Part model, mm, in its own coordinate system. Face numbers are marked on the shaded views. Round coordinates to 2 decimals unless told otherwise and drop trailing zeros. Order: outer loops, then holes, each group sorted by start corner. A loop starts at its lowest first (then second) coordinate and runs counter-clockwise, first axis right, second up. Notation, with made-up numbers: M -25,-31.75 L 10,-31.75 A28 cw 10,-5.75 Z; hole C 3,-23 d2. An arc over 180 degrees is marked long. Write each question's results on one line, items separated by ' | '. Start each with the question number.
1. Drop flat-ended pins along their axis: pin 1 Ø16 at (x, y) = (31.5, 37) entering from +Z; pin 2 Ø10.5 at (x, y) = (0, 57) entering from -Z; pin 3 Ø5 at (y, z) = (50.5, 1.5) entering from -X. Give the stop position or say it passes through.
2. Two-plate mould, pull along X, no slides. Class the marked faces 1, 2 and 3: +X half, -X half, draft (parallel to the pull), parting line (faces both ways), or undercut.
3. Probe L1, parallel to Y at x = 42.5, z = 7; L2, parallel to Y at x = 0, z = 4.4; L3, parallel to X at y = 57, z = 4.1. List the from-to ranges inside material, lowest first. Write a range as [from, to].
4. Band-saw the part on A-A, the plane z = 9.5. List the corners of the cut face in (x, y).
5. Band-saw the part on B-B, the plane x = 1.5. List the corners of the cut face in (y, z), then the cut area to 3 significant figures.
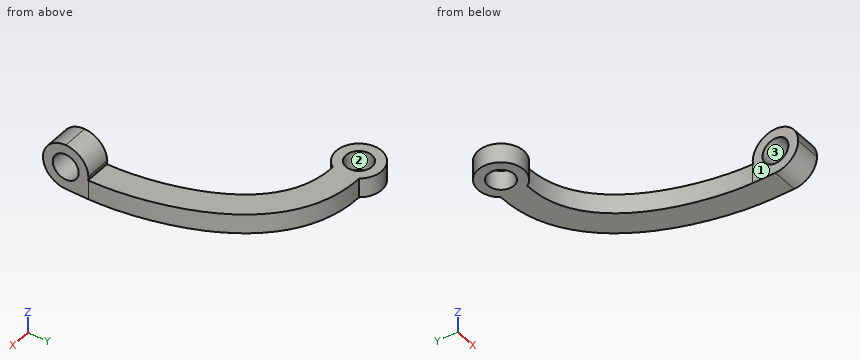
```python
from build123d import *
from OCP.BRepAlgoAPI import BRepAlgoAPI_Cut
from OCP.TopTools import TopTools_ListOfShape

# Parameters (mm, degrees)
ESBO_O1_R                = 4
RESSALTO_EXTRUS_O1_DEPTH = 14
ESBO_O2_R                = 4
CORTE_EXTRUS_O1_DEPTH    = 85.267431587


with BuildPart() as part:
    # Esboço1 → Ressalto-extrusão1 (new body)
    with BuildSketch(Plane.XY):
        with BuildLine():
            Line((46, -7), (46, 6.995688759))
            add(Edge.make_bspline(
                [(5.650259544, 61.132138319), (6.660650147, 61.155575151), (8.710848107, 61.120789853), (12.578892548, 60.727605083), (17.127930578, 59.655790613), (22.040205616, 57.539349047), (26.394344624, 54.722364625), (30.19261077, 51.343572081), (34.558581899, 46.260896731), (38.815468688, 39.112541001), (41.760696394, 31.545459809), (43.470535674, 25.587286464), (44.459557745, 21.252306014), (45.183880004, 17.135758602), (45.589217997, 13.957943213), (45.8071763, 11.605329402), (45.920450747, 9.949575993), (45.986308659, 8.391657602), (46.000256085, 7.470883976), (46, 6.995688759)],
                knots=[0, 0, 0, 0, 0.03125, 0.0625, 0.125, 0.1875, 0.25, 0.3125, 0.375, 0.5, 0.625, 0.6875, 0.75, 0.8125, 0.875, 0.90625, 0.9375, 0.96875, 1, 1, 1, 1], degree=3))
            ThreePointArc((5.650259544, 61.132138319), (-6.998117599, 56.837672963), (5.835776158, 53.134289634))
            add(Edge.make_bspline(
                [(5.835776158, 53.134289634), (6.238188643, 53.143623919), (7.052270041, 53.146185942), (8.608930463, 53.086843267), (10.474039614, 52.897553491), (12.577068171, 52.49932445), (15.220765339, 51.755589596), (18.249448664, 50.451415), (21.515264324, 48.342822315), (24.453790354, 45.735335437), (27.957095233, 41.667286815), (31.567422767, 35.644835437), (34.179252288, 28.956801958), (35.718249768, 23.595597215), (36.614783762, 19.667281612), (37.272272941, 15.930397286), (37.638098577, 13.059067768), (37.83252613, 10.960084825), (37.932188748, 9.497611194), (37.979377076, 8.387903873), (37.997359238, 7.565341164), (38.000104404, 7.191578727), (38.000001162, 7)],
                knots=[0, 0, 0, 0, 0.015625, 0.03125, 0.0625, 0.09375, 0.125, 0.1875, 0.25, 0.3125, 0.375, 0.5, 0.625, 0.6875, 0.75, 0.8125, 0.875, 0.90625, 0.9375, 0.96875, 0.984375, 1, 1, 1, 1], degree=3))
            Line((38.000001162, 7), (38.000001162, -7))
            Line((38.000001162, -7), (46, -7))
        make_face()
        with Locations((0, 57)):
            Circle(ESBO_O1_R, mode=Mode.SUBTRACT)
    extrude(amount=RESSALTO_EXTRUS_O1_DEPTH)


with BuildPart() as corte_extrus_o1_tool:
    # Esboço2 → Corte-extrusão1 (new, through all)
    with BuildSketch(Plane(origin=(46, 0, 0), x_dir=(0, 0, -1), z_dir=(1, 0, 0))):
        with BuildLine():
            ThreePointArc((-7, -7), (-11.949747468, -4.949747468), (-14, 0))
            Line((-14, 0), (-14, -7))
            Line((-14, -7), (-7, -7))
        make_face()
        with BuildLine():
            Line((-7.245639543, 6.995688759), (-14, 6.995688759))
            Line((-14, 6.995688759), (-14, 0))
            ThreePointArc((-14, 0), (-12.035845351, 4.862125214), (-7.245639543, 6.995688759))
        make_face()
        with Locations((-7, 0)):
            Circle(ESBO_O2_R)
        with BuildLine():
            Line((0, -7), (0, 0))
            ThreePointArc((0, 0), (-2.050252532, -4.949747468), (-7, -7))
            Line((-7, -7), (0, -7))
        make_face()
        with BuildLine():
            Line((-6, 6.92820323), (-6, 6.995688759))
            Line((-6, 6.995688759), (-6.754360457, 6.995688759))
            ThreePointArc((-6.754360457, 6.995688759), (-6.37626685, 6.972155833), (-6, 6.92820323))
        make_face()
        with BuildLine():
            Line((-6, 6.995688759), (-6, 64))
            Line((-6, 64), (-14, 64))
            Line((-14, 64), (-14, 6.995688759))
            Line((-14, 6.995688759), (-7.245639543, 6.995688759))
            ThreePointArc((-7.245639543, 6.995688759), (-7, 7), (-6.754360457, 6.995688759))
            Line((-6.754360457, 6.995688759), (-6, 6.995688759))
        make_face()
    extrude(amount=-CORTE_EXTRUS_O1_DEPTH)


with BuildPart() as part_1:
    add(part.part)

    # Corte-extrusão1: cut by corte_extrus_o1_tool, with a tolerance
    corte_extrus_o1_stock = TopTools_ListOfShape()
    corte_extrus_o1_stock.Append(part_1.part.wrapped)
    corte_extrus_o1_tools = TopTools_ListOfShape()
    corte_extrus_o1_tools.Append(corte_extrus_o1_tool.part.wrapped)
    corte_extrus_o1_cut = BRepAlgoAPI_Cut()
    corte_extrus_o1_cut.SetArguments(corte_extrus_o1_stock)
    corte_extrus_o1_cut.SetTools(corte_extrus_o1_tools)
    corte_extrus_o1_cut.SetFuzzyValue(0.00001)
    corte_extrus_o1_cut.Build()
    add(Compound.cast(corte_extrus_o1_cut.Shape()).solids(), mode=Mode.REPLACE)


with BuildPart() as corte_extrus_o1_kept_piece:
    # of the separate pieces the step leaves, the one the design keeps (corte_extrus_o1_pieces_kept)
    add(part_1.part.solids().sort_by_distance((46, 0, 0))[0])


solid = corte_extrus_o1_kept_piece.part
```
Solution:
1) pin 1: z = 6 | pin 2: z = 0 | pin 3: x = -5.74
2) face 1: -X half | face 2: undercut | face 3: draft
3) L1: [-7, -4], [4, 7] | L2: [50, 53], [61, 64] | L3: [-7, -4], [4, 22.71]
4) outline: M 38,-6.54 L 46,-6.54 L 46,-3.12 L 38,-3.12 Z; M 38,3.12 L 46,3.12 L 46,6.54 L 38,6.54 Z
5) outline: M 50.16,0 L 53.29,0 L 53.29,6 L 50.16,6 Z; M 60.71,0 L 63.84,0 L 63.84,6 L 60.71,6 Z | area: 37.6 mm^2
